```python
from build123d import *

# Parameters (mm, degrees)
SKETCH4_R                         = 14.2875
CUT_EXTRUDE1_DEPTH                = 406.190469782
CIRPATTERN2_COUNT                 = 28
CIRPATTERN3_COUNT                 = 12
CIRPATTERN4_COUNT                 = 4
CIRPATTERN5_COUNT                 = 56
F_1_2_13_TAPPED_HOLE4_D           = 10.71626
F_1_2_13_TAPPED_HOLE4_DEPTH       = 35.052
F_1_2_13_TAPPED_HOLE4_CSINK_D     = 13.97
F_1_2_13_TAPPED_HOLE4_CSINK_ANGLE = 100
F_1_2_13_TAPPED_HOLE4_TIP         = 3.219489309


with BuildPart() as part:
    # Sketch1 → Revolve1 (revolve)
    with BuildSketch(Plane.XY, mode=Mode.PRIVATE) as revolve1_sk:
        with BuildLine():
            Line((-4.7752, 67.5132), (-4.7752, 180.9496))
            Line((-4.7752, 180.9496), (0, 180.9496))
            Line((0, 180.9496), (0, 228.9937))
            Line((0, 228.9937), (-4.7752, 228.9937))
            Line((-4.7752, 228.9937), (-4.7752, 281.051))
            Line((-4.7752, 281.051), (32.512, 281.051))
            Line((32.512, 281.051), (32.512, 231.3686))
            Line((32.512, 231.3686), (51.6128, 231.3686))
            Line((51.6128, 231.3686), (51.6128, 217.9066))
            Line((51.6128, 217.9066), (73.9648, 217.9066))
            Line((73.9648, 217.9066), (73.9648, 67.6275))
            Line((73.9648, 67.6275), (51.892823931, 33.9957528))
            ThreePointArc((51.892823931, 33.9957528), (50.746661337, 32.943911593), (49.238413158, 32.5628))
            Line((49.238413158, 32.5628), (47.625, 32.5628))
            Line((47.625, 32.5628), (47.625, 67.5132))
            Line((47.625, 67.5132), (-4.7752, 67.5132))
        make_face()
    revolve(revolve1_sk.sketch.rotate(Axis((0, 0, 0), (1, 0, 0)), 90), axis=Axis((0, 0, 0), (1, 0, 0)))

    # Sketch4 → Cut-Extrude1 (cut, through all)
    with BuildSketch(Plane.ZY.offset(4.7752)):
        with Locations((28.972111579, 257.135466548)):
            Circle(SKETCH4_R)
    cut_extrude1 = extrude(amount=-CUT_EXTRUDE1_DEPTH, mode=Mode.SUBTRACT)

    # CirPattern2: Cut-Extrude1 ×28 about axis
    cirpattern2_axis = Axis((0, 0, 0), (1, 0, 0))
    for i in range(1, CIRPATTERN2_COUNT):
        add(cut_extrude1.rotate(cirpattern2_axis, i * 360 / CIRPATTERN2_COUNT), mode=Mode.SUBTRACT)

    # Sketch8 → 3/4-10 Tapped Hole1 (revolve, cut)
    with BuildSketch(Plane(origin=(0, 199.3429424, 53.413780433), x_dir=(0, 0, 1), z_dir=(0, 1, 0))):
        Polygon((0, 0), (0, 30.407416175), (8.33374, 25.4), (8.33374, 1.82626), (10.16, 0), align=None)
    f_3_4_10_tapped_hole1 = revolve(axis=Axis((-6.35, 199.3429424, 53.413780433), (1, 0, 0)), mode=Mode.SUBTRACT)

    # CirPattern3: 3/4-10 Tapped Hole1 ×12 about axis
    cirpattern3_axis = Axis((0, 0, 0), (1, 0, 0))
    for i in range(1, CIRPATTERN3_COUNT):
        add(f_3_4_10_tapped_hole1.rotate(cirpattern3_axis, i * 360 / CIRPATTERN3_COUNT), mode=Mode.SUBTRACT)

    # Sketch10 → 7/8-9 Tapped Hole1 (revolve, cut)
    with BuildSketch(Plane(origin=(-4.7752, 67.172315786, 67.172315786), x_dir=(0, 0, 1), z_dir=(0, 1, 0))):
        Polygon((0, 0), (0, 31.242239902), (9.72312, 25.4), (9.72312, 2.02438), (11.7475, 0), align=None)
    f_7_8_9_tapped_hole1 = revolve(axis=Axis((-11.1252, 67.172315786, 67.172315786), (1, 0, 0)), mode=Mode.SUBTRACT)

    # CirPattern4: 7/8-9 Tapped Hole1 ×4 about axis
    cirpattern4_axis = Axis((0, 0, 0), (1, 0, 0))
    for i in range(1, CIRPATTERN4_COUNT):
        add(f_7_8_9_tapped_hole1.rotate(cirpattern4_axis, i * 360 / CIRPATTERN4_COUNT), mode=Mode.SUBTRACT)

    # Sketch21 → Tap Drill for 3/8-16 Tap1 (revolve, cut)
    with BuildSketch(Plane(origin=(-4.7752, 162.844517689, 201.096231852), x_dir=(0, 0, 1), z_dir=(0, 1, 0))):
        Polygon((0, 0), (0, 43.024665582), (3.96875, 40.64), (3.96875, 0.635), (4.60375, 0), align=None)
    tap_drill_for_3_8_16_tap1 = revolve(axis=Axis((-11.1252, 162.844517689, 201.096231852), (1, 0, 0)), mode=Mode.SUBTRACT)

    # CirPattern5: Tap Drill for 3/8-16 Tap1 ×56 about axis, 52 skipped
    cirpattern5_axis = Axis((0, 0, 0), (-1, 0, 0))
    add([tap_drill_for_3_8_16_tap1.rotate(cirpattern5_axis, i * 360 / CIRPATTERN5_COUNT) for i in range(1, CIRPATTERN5_COUNT) if i not in (1, 2, 3, 4, 5, 6, 7, 8, 9, 10, 11, 12, 13, 14, 15, 17, 18, 19, 20, 21, 22, 23, 24, 25, 26, 27, 29, 30, 31, 32, 33, 34, 35, 36, 37, 38, 39, 40, 41, 42, 43, 45, 46, 47, 48, 49, 50, 51, 52, 53, 54, 55)], mode=Mode.SUBTRACT)

    # 1/2-13 Tapped Hole4
    with Locations(Plane(origin=(12.5984, 281.051, 0), x_dir=(0, 0, 1), z_dir=(0, 1, 0))):
        with Locations((0, 0)):
            CounterSinkHole(F_1_2_13_TAPPED_HOLE4_D / 2, F_1_2_13_TAPPED_HOLE4_CSINK_D / 2, depth=F_1_2_13_TAPPED_HOLE4_DEPTH, counter_sink_angle=F_1_2_13_TAPPED_HOLE4_CSINK_ANGLE)
            with Locations((0, 0, -(F_1_2_13_TAPPED_HOLE4_DEPTH + F_1_2_13_TAPPED_HOLE4_TIP / 2))):  # 118° drill point
                Cone(0, F_1_2_13_TAPPED_HOLE4_D / 2, F_1_2_13_TAPPED_HOLE4_TIP, mode=Mode.SUBTRACT)


solid = part.part
```
Model file for the job. Use its own axes, mm. A direction names the side the tool comes from. Give positions to 0.01 mm unless a question says otherwise; leave off trailing zeros. Loops run counter-clockwise (first coordinate to the right, second up) from the corner with the lowest first, then second, coordinate; pieces in that order, holes last. Notation, with made-up numbers: (-19, 34) - (32, 34) arc R21 ccw to (32, 62) - close; hole circle Ø7 at (6.25, 51). An arc over 180 degrees is marked (long way). One line per item, written item: value. Start each with the question number.
1. Which spindle directions (+Z, -Z, +X, -X, +Y, -Y) get a long thin tool onto all of the face, cutting with end or side? Do faces 1 (the cylindrical face through (13.61, -190.35, 195.21)), 2 (the cylindrical face through (-2.354, -54.352, 172.594)). Say none if no direction does.
2. Pull direction Y, two halves, no side cores. Call faces 3 (the cylindrical face through (21.058, 41.081, -53.576)), 4 (the flat face through (-4.775, 78, 3)), 5 (the cylindrical face through (62.945, -65.453, 207.844)): pulls with the +Y half, pulls with the -Y half, needs draft (parallel to the pull), parting line crosses it, or undercut.
3. Probe L1, parallel to Y at x = -1.1, z = 0; L2, parallel to Z at x = 11, y = -51.5; L3, parallel to Y at x = 18, z = -29.5. List the from-to ranges inside material, lowest first. Write a range as from..to.
4. Slice it at B-B (y = 111). List the corners of the cut face in (x, z).
5. Pin check, flat tips, straight feed: pin 1 (10 mm diameter, centred on y = -53.41, z = 199.34, fed in from -X); pin 2 (10.5 mm diameter, centred on y = 159.82, z = -203.51, fed in from +X); pin 3 (2 mm diameter, centred on x = 17, z = 183.5, fed in from -Y). Stop position of each tip, or through.
Solution:
1. face 1: +X, -X
1. face 2: -X
2. face 3: undercut
2. face 4: needs draft
2. face 5: parting line crosses it
3. L1: y = -281.05..-228.99, -180.95..-67.51, 67.51..180.95, 228.99..281.05
3. L2: z = -276.29..-207.45, -191.23..-43.66, 43.66..191.23, 207.45..276.29
3. L3: y = -279.5..-271.41, -242.86..-60.73, 60.73..242.86, 271.41..279.5
4. outline: (-4.78, -258.2) - (32.51, -258.2) - (32.51, -203) - (51.61, -203) - (51.61, -187.52) - (73.96, -187.52) - (73.96, 187.52) - (51.61, 187.52) - (51.61, 203) - (32.51, 203) - (32.51, 258.2) - (-4.78, 258.2) - (-4.78, 200.29) - (0, 200.29) - (0, 142.9) - (-4.78, 142.9) - (-4.78, -142.9) - (0, -142.9) - (0, -200.29) - (-4.78, -200.29) - close
5. pin 1: stops at x = 27.4
5. pin 2: stops at x = 32.51
5. pin 3: stops at y = -213.74
